```python
from build123d import *

# Parameters (mm, degrees)
SKETCH_2_W               = 109.92
SKETCH_2_H               = 76
EXTRUDE_1_DEPTH          = 10
CUT_EXTRUDE_1_DEPTH      = 5
SKETCH_4_R               = 2
CUT_EXTRUDE_2_DEPTH      = 92.808295873
SKETCH_5_W               = 109.92
SKETCH_5_H               = 6
EXTRUDE_2_DEPTH          = 25
CUT_EXTRUDE_3_DEPTH      = 104.340627651
CUT_EXTRUDE_3_DEPTH_BACK = 104.340627651
SKETCH_7_R               = 2.1
SKETCH_9_R               = 2.1
CUT_EXTRUDE_4_DEPTH      = 96.019804204
CUT_EXTRUDE_5_DEPTH      = 5
EXTRUDE_3_DEPTH          = 35
FILLET_1_R               = 2
EXTRUDE_4_DEPTH          = 4


with BuildPart() as part:
    # 草圖2 → 填料-伸長1 (new body)
    with BuildSketch(Plane.XY):
        with Locations((12.52544527, 24.044160626)):
            Rectangle(SKETCH_2_W, SKETCH_2_H)
    extrude(amount=EXTRUDE_1_DEPTH)

    # 草圖3 → 除料-伸長1 (cut)
    with BuildSketch(Plane.XY.offset(10)):
        with BuildLine():
            Line((67.48544527, -6.055839374), (67.48544527, 54.144160626))
            Line((67.48544527, 54.144160626), (61.24181631, 50.538464901))
            ThreePointArc((61.24181631, 50.538464901), (61.408690367, 50.105080914), (61.46544527, 49.644160626))
            ThreePointArc((61.46544527, 49.644160626), (60.088104264, 47.81746208), (57.95299519, 48.639170705))
            Line((57.95299519, 48.639170705), (55.48544527, 47.214160626))
            Line((55.48544527, 47.214160626), (55.48544527, 0.874160626))
            Line((55.48544527, 0.874160626), (57.95299519, -0.550849453))
            ThreePointArc((57.95299519, -0.550849453), (60.088104264, 0.270859171), (61.46544527, -1.555839374))
            ThreePointArc((61.46544527, -1.555839374), (61.408690367, -2.016759663), (61.24181631, -2.45014365))
            Line((61.24181631, -2.45014365), (67.48544527, -6.055839374))
        make_face()
    extrude(amount=-CUT_EXTRUDE_1_DEPTH, mode=Mode.SUBTRACT)

    # 草圖4 → 除料-伸長2 (cut, through all)
    with BuildSketch(Plane.XY.offset(5)):
        with Locations((59.56544527, 41.644160626)):
            Circle(SKETCH_4_R)
        with Locations((59.56544527, 33.644160626)):
            Circle(SKETCH_4_R)
        with Locations((59.56544527, 6.444160626)):
            Circle(SKETCH_4_R)
        with Locations((59.56544527, 14.444160626)):
            Circle(SKETCH_4_R)
    extrude(amount=-CUT_EXTRUDE_2_DEPTH, mode=Mode.SUBTRACT)

    # 草圖5 → 填料-伸長2 (add)
    with BuildSketch(Plane.XY.offset(10)):
        with Locations((12.52544527, -10.955839374)):
            Rectangle(SKETCH_5_W, SKETCH_5_H)
        with Locations((12.52544527, 59.044160626)):
            Rectangle(SKETCH_5_W, SKETCH_5_H)
    extrude(amount=EXTRUDE_2_DEPTH)

    # 草圖7 → 除料-伸長3 (cut, two sides: drawn at the far end of the back side and taken through both)
    with BuildSketch(Plane(origin=(0, -7.955839374, 0), x_dir=(1, 0, 0), z_dir=(0, 1, 0)).offset(-CUT_EXTRUDE_3_DEPTH_BACK)):
        with Locations(Location((-36.43455473, -18, 0), (0, 0, 270))):
            Circle(SKETCH_7_R)
        with Locations(Location((-36.43455473, -26, 0), (0, 0, 270))):
            Circle(SKETCH_7_R)
    extrude(amount=CUT_EXTRUDE_3_DEPTH + CUT_EXTRUDE_3_DEPTH_BACK, mode=Mode.SUBTRACT)

    # 草圖9 → 除料-伸長4 (cut, through all)
    with BuildSketch(Plane.XY.offset(10)):
        with Locations((-36.43455473, 0.044160626)):
            Circle(SKETCH_9_R)
        with Locations((-36.43455473, 8.044160626)):
            Circle(SKETCH_9_R)
        with Locations((-36.43455473, 16.044160626)):
            Circle(SKETCH_9_R)
        with Locations((-36.43455473, 24.044160626)):
            Circle(SKETCH_9_R)
        with Locations((-36.43455473, 32.044160626)):
            Circle(SKETCH_9_R)
        with Locations((-36.43455473, 40.044160626)):
            Circle(SKETCH_9_R)
        with Locations((-36.43455473, 48.044160626)):
            Circle(SKETCH_9_R)
    extrude(amount=-CUT_EXTRUDE_4_DEPTH, mode=Mode.SUBTRACT)

    # 草圖10 → 除料-伸長5 (cut)
    with BuildSketch(Plane(origin=(0, 0, 0), x_dir=(-1, 0, 0), z_dir=(0, 0, -1))):
        with BuildLine():
            Line((32.43455473, 0.044160626), (32.43455473, 48.044160626))
            ThreePointArc((32.43455473, 48.044160626), (36.43455473, 52.044160626), (40.43455473, 48.044160626))
            Line((40.43455473, 48.044160626), (40.43455473, 0.044160626))
            ThreePointArc((40.43455473, 0.044160626), (36.43455473, -3.955839374), (32.43455473, 0.044160626))
        make_face()
    extrude(amount=-CUT_EXTRUDE_5_DEPTH, mode=Mode.SUBTRACT)

    # 草圖12 → 填料-伸長3 (add)
    with BuildSketch(Plane.XY.offset(35)):
        Polygon((17.670490694, 69.044160626), (13.629038809, 62.044160626), (18.247840963, 62.044160626), (21.134592309, 67.044160626), align=None)
        Polygon((24.598693924, 65.044160626), (22.866643116, 62.044160626), (27.48544527, 62.044160626), (28.062795539, 63.044160626), align=None)
        Polygon((18.247840963, -13.955839374), (13.629038809, -13.955839374), (17.670490694, -20.955839374), (21.134592309, -18.955839374), align=None)
        Polygon((27.48544527, -13.955839374), (22.866643116, -13.955839374), (24.598693924, -16.955839374), (28.062795539, -14.955839374), align=None)
    extrude(amount=-EXTRUDE_3_DEPTH)

    # 圓角1
    fillet_1_edges = [part.edges().sort_by_distance(p)[0] for p in [
        (12.52544527, 56.044160626, 10),
        (12.52544527, -7.955839374, 10),
        (-42.43455473, 62.044160626, 17.5),
        (-42.43455473, -13.955839374, 17.5),
        (-42.43455473, 24.044160626, 0),
        (-14.40275796, -13.955839374, 0),
        (15.649764752, -17.455839374, 0),
        (15.649764752, 65.544160626, 0),
        (13.629038809, -13.955839374, 17.5),
        (13.629038809, 62.044160626, 17.5),
        (-14.40275796, 62.044160626, 0),
    ]]
    fillet(fillet_1_edges, radius=FILLET_1_R - 0.0001)  # a hair under: the kernel refuses the full size

    # 草圖13 → 填料-伸長4 (add)
    with BuildSketch(Plane(origin=(0, 0, 0), x_dir=(-1, 0, 0), z_dir=(0, 0, -1))):
        Polygon((-21.134592309, -18.955839374), (-24.598693924, -16.955839374), (-22.866643116, -13.955839374), (-18.247840963, -13.955839374), align=None)
        Polygon((-22.866643116, 62.044160626), (-24.598693924, 65.044160626), (-21.134592309, 67.044160626), (-18.247840963, 62.044160626), align=None)
    extrude(amount=-EXTRUDE_4_DEPTH)


solid = part.part
```
Model file for the job. Use its own axes, mm. A direction names the side the tool comes from. Give positions to 0.01 mm unless a question says otherwise; leave off trailing zeros. Write each loop counter-clockwise with the first axis right and the second up, starting at its lowest first coordinate (ties: lowest second). Pieces come first, ordered by that corner, then holes. Notation, with made-up numbers: (38.5, -40) -> (57.5, -40) arc R30 cw to (57.5, -1) -> close; hole circle Ø6 at (12.25, 10.5). An arc over 180 degrees is marked (long way). Use CSV: the item, a comma, the result in double quotes. Start each with the question number.
1) Cut at D-D on z = 7. Count the separate pieces of the cut face and the enclosed holes in it, plus the area to 3 significant figures.
2) Cut at C-C on x = -26. List the corners of the cut face in (y, z), plus the area to 3 significant figures.
3) Pin check, flat tips, straight feed: P1, Ø1.5, axis at x = 23, y = 64, coming from the +Z side; P2, Ø7, axis at x = -10.5, z = 22, coming from the +Y side; P3, Ø5, axis at x = 36.5, y = 12.5, coming from the +Z side. Stop position of each tip, or through.
4) Drill centre lines: L1, parallel to Y at x = 22.5, z = 18; L2, parallel to X at y = 57.75, z = 18; L3, parallel to Z at x = -10, y = -0.5. Where is each one in solid material? Low to high.
5) Cut at B-B on x = 38. List the corners of the cut face in (y, z).
6) Cut at A-A on z = 22.5. List the corners of the cut face in (x, y), plus the area to 3 significant figures.
7) Tool access for faces 4 (the flat face through (23.745, 63.565, 19.717)), 5 (the cylindrical face through (-36.523, -3.955, 2.465)), 6 (the flat face through (23.7, -15.4, 19.7)): list every direction of +Z, -Z, +X, -X, +Y, -Y with a clear straight run to the whole face (end or side of a thin tool).
8) Two-plate mould, pull along X, no slides. Class faces 1 (the cylindrical face through (-34.35, -11, 17.73)), 2 (the flat face through (47, -13.956, 17)), 3 (the flat face through (64.32, -4.23, 7.54)): released by +X, released by -X, zero draft, split by the parting line, or undercut.
Final values:
1,separate pieces,"1"
1,enclosed holes,"7"
1,area,"7,700 mm2"
2,outline,"(-13.96, 2) arc R2 ccw to (-11.96, 0) -> (60.04, 0) arc R2 ccw to (62.04, 2) -> (62.04, 35) -> (56.04, 35) -> (56.04, 12) arc R2 cw to (54.04, 10) -> (-5.96, 10) arc R2 cw to (-7.96, 12) -> (-7.96, 35) -> (-13.96, 35) -> close"
2,area,"1,060 mm2"
3,P1,"stops at z = 4"
3,P2,"stops at y = 62.04"
3,P3,"stops at z = 10"
4,L1,"y = -13.96 to -7.96, 56.04 to 62.04"
4,L2,"x = -42.43 to -38.53, -34.33 to 67.49"
4,L3,"z = 0 to 10"
5,outline,"(-13.96, 0) -> (62.04, 0) -> (62.04, 35) -> (56.04, 35) -> (56.04, 12) arc R2 cw to (54.04, 10) -> (-5.96, 10) arc R2 cw to (-7.96, 12) -> (-7.96, 35) -> (-13.96, 35) -> close"
6,outline,"(-42.43, -11.96) arc R2 ccw to (-40.43, -13.96) -> (12.47, -13.96) arc R2 cw to (14.21, -14.96) -> (17.67, -20.96) -> (21.13, -18.96) -> (18.25, -13.96) -> (22.87, -13.96) -> (24.6, -16.96) -> (28.06, -14.96) -> (27.49, -13.96) -> (67.49, -13.96) -> (67.49, -7.96) -> (-42.43, -7.96) -> close; (-42.43, 56.04) -> (67.49, 56.04) -> (67.49, 62.04) -> (27.49, 62.04) -> (28.06, 63.04) -> (24.6, 65.04) -> (22.87, 62.04) -> (18.25, 62.04) -> (21.13, 67.04) -> (17.67, 69.04) -> (14.21, 63.04) arc R2 cw to (12.47, 62.04) -> (-40.43, 62.04) arc R2 ccw to (-42.43, 60.04) -> close"
6,area,"1,390 mm2"
7,face 4,"+Z, +Y"
7,face 5,"-Z"
7,face 6,"+Z, -Y"
8,face 1,"undercut"
8,face 2,"zero draft"
8,face 3,"released by +X"
